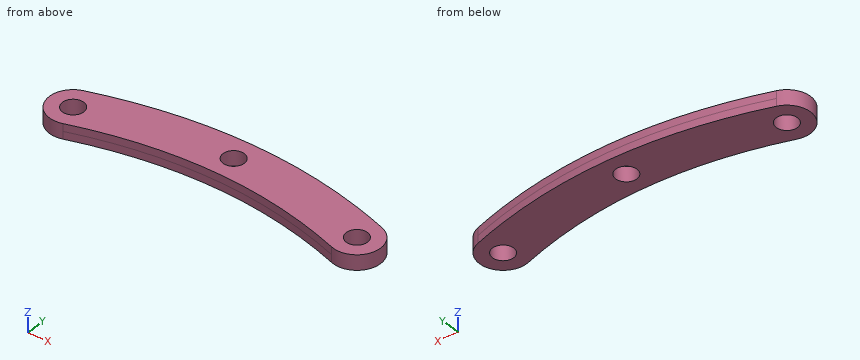
```python
from build123d import *

# Parameters (mm, degrees)
BOSS_EXTRUDE1_DEPTH  = 1.5875
M4_CLEARANCE_HOLE1_D = 4.5


with BuildPart() as part:
    # Sketch1 → Boss-Extrude1 (new body, symmetric)
    with BuildSketch(Plane.XY):
        with BuildLine():
            ThreePointArc((-28.41886117, -9.74341649), (-34.74341649, -6.58113883), (-31.58113883, -0.25658351))
            add(Edge.make_bspline(
                [(-31.58113883, -0.25658351), (-19.788717071, 3.678862016), (0, 5.330284496), (19.788717071, 3.678862016), (31.58113883, -0.25658351)],
                knots=[0, 0, 0, 0.375, 0.625, 1, 1, 1], degree=2))
            ThreePointArc((31.58113883, -0.25658351), (34.74341649, -6.58113883), (28.41886117, -9.74341649))
            add(Edge.make_bspline(
                [(-28.41886117, -9.74341649), (-17.711282929, -6.178862016), (0, -4.705284496), (17.711282929, -6.178862016), (28.41886117, -9.74341649)],
                knots=[0, 0, 0, 0.375, 0.625, 1, 1, 1], degree=2))
        make_face()
    extrude(amount=BOSS_EXTRUDE1_DEPTH, both=True)

    # M4 Clearance Hole1 (through all)
    with Locations(Plane.XY.offset(1.5875)):
        with Locations((-30, -5), (30, -5), (0, 0)):
            Hole(M4_CLEARANCE_HOLE1_D / 2)


solid = part.part
```
Model file for the job. Use its own axes, mm. Coordinates: 2 decimals unless noted, no trailing zeros. Return JSON: item names as keys, results as strings. Group by question number.
1) Flat gauge pins, fed straight in: P1, Ø1, axis at y = -6, z = 0.5, coming from the +X side; P2, Ø1, axis at x = -1, z = 0.5, coming from the +Y side. Where does each tip first touch, or does it go through?
2) Probe line 1 (X direction, y = -4.75, z = 1.3); line 2 (Y direction, x = 0, z = -0.7); line 3 (Y direction, x = 2, z = 1.15). List the from-to ranges inside material, lowest first. Write a range as from..to.
3) Saw through at A-A, the plane z = 0.7. Count the separate pieces of the cut face and the enclosed holes in it, plus the area to 3 significant figures.
Values found:
{
 "1": {"P1": "stops at x = 34.97", "P2": "stops at y = 5"},
 "2": {"line 1": "x = -34.99..-32.24, -27.76..27.76, 32.24..34.99", "line 2": "y = -5..-2.25, 2.25..5", "line 3": "y = -5.02..-1.03, 1.03..4.98"},
 "3": {"separate pieces": "1", "enclosed holes": "3", "area": "642 mm²"}
}
